from build123d import *

# Parameters (mm, degrees)
SKETCH1_W                      = 22.5
SKETCH1_H                      = 20
BOSS_EXTRUDE1_DEPTH            = 3.175
CBORE_FOR_M2_SHCS1_D           = 2.2
CBORE_FOR_M2_SHCS1_CBORE_D     = 4.4
CBORE_FOR_M2_SHCS1_CBORE_DEPTH = 2
TAP_DRILL_FOR_M2X0_4_TAP1_D    = 1.6
TAP_DRILL_FOR_M2X0_4_TAP2_D    = 1.6
FILLET1_SIZE                   = 1


with BuildPart() as part:
    # Sketch1 → Boss-Extrude1 (new body)
    with BuildSketch(Plane.XY):
        Rectangle(SKETCH1_W, SKETCH1_H)
    extrude(amount=BOSS_EXTRUDE1_DEPTH)

    # CBORE for M2 SHCS1 (through all)
    with Locations(Plane.XY.offset(3.175)):
        with Locations((4, 6), (-4, -6), (-4, 6), (4, -6)):
            CounterBoreHole(CBORE_FOR_M2_SHCS1_D / 2, CBORE_FOR_M2_SHCS1_CBORE_D / 2, CBORE_FOR_M2_SHCS1_CBORE_DEPTH)

    # Tap Drill for M2x0.4 Tap1 (through all)
    with Locations(Plane(origin=(0, 10, 0), x_dir=(1, 0, 0), z_dir=(0, 1, 0))):
        with Locations((8, -1.5875), (-8, -1.5875)):
            Hole(TAP_DRILL_FOR_M2X0_4_TAP1_D / 2)

    # Tap Drill for M2x0.4 Tap2 (through all)
    with Locations(Plane.XY.offset(3.175)):
        with Locations((0, 0), (-4.949747468, 0), (0, -4.949747468), (4.949747468, 0), (0, 4.949747468)):
            Hole(TAP_DRILL_FOR_M2X0_4_TAP2_D / 2)

    # Fillet1
    fillet1_edges = [part.edges().sort_by_distance(p)[0] for p in [
        (11.25, -10, 1.5875),
        (-11.25, -10, 1.5875),
        (-11.25, 10, 1.5875),
        (11.25, 10, 1.5875),
    ]]
    chamfer(fillet1_edges, length=FILLET1_SIZE)


solid = part.part
Geometry: final body of the model. Coordinates: model frame, mm. A direction names the side the tool comes from. Round coordinates to 2 decimals unless told otherwise and drop trailing zeros. Order: outer loops, then holes, each group sorted by start corner. A loop starts at its lowest first (then second) coordinate and runs counter-clockwise, first axis right, second up. Notation, with made-up numbers: (-32, -21) - (-18, -21) arc R34 cw to (-18, 15) - close; hole circle Ø1 at (35, 5.25). An arc over 180 degrees is marked (long way). Write each question's results on one line, items separated by ' | '.
Item 1: First-contact query: pin 1 Ø1.3 at (x, y) = (-3.5, 6.5) entering from +Z (3 decimals); pin 2 Ø1 at (x, y) = (4.95, 0) entering from +Z. Flat tips, straight axial feed; report the tip coordinate or a pass-through.
Completed:
pin 1: z = 1.175 | pin 2: through
Item 2: Section B-B, the plane x = -8. Return the cut outline in (y, z) (1 decimal).
Completed:
outline: (-10, 0) - (10, 0) - (10, 0.8) - (-10, 0.8) - close; (-10, 2.4) - (10, 2.4) - (10, 3.2) - (-10, 3.2) - close
Item 3: Reachability of faces 4 (the flat face through (10.76, -9.49, 1.57)), 5 (the cylindrical face through (-1.9, 6.66, 2.19)) from +Z, -Z, +X, -X, +Y, -Y: full face, straight path, thin tool, end or side. Return the list, or none.
Completed:
face 4: +Z, -Z, +X, -Y | face 5: +Z
Item 4: Section D-D, the plane x = -3.5. Return the cut outline in (y, z) (3 decimals), and give its area (3 significant figures).
Completed:
outline: (-10, 0) - (-6.98, 0) - (-6.98, 1.175) - (-8.142, 1.175) - (-8.142, 3.175) - (-10, 3.175) - close; (-5.02, 0) - (5.02, 0) - (5.02, 1.175) - (3.858, 1.175) - (3.858, 3.175) - (-3.858, 3.175) - (-3.858, 1.175) - (-5.02, 1.175) - close; (6.98, 0) - (10, 0) - (10, 3.175) - (8.142, 3.175) - (8.142, 1.175) - (6.98, 1.175) - close | area: 41.8 mm^2
Item 5: Section A-A, the plane y = 0. State how many separate pieces and enclosed holes the cut face has, and give its area (3 significant figures).
Completed:
separate pieces: 4 | enclosed holes: 2 | area: 52.2 mm^2
Item 6: Material intervals for line 1 along Y through (x, z) = (0, 0.9); line 2 along Y through (x, z) = (4, 0.3); line 3 along Y through (x, z) = (4, 2.65), sorted ascending. Write a range as [from, to].
Completed:
line 1: [-10, -5.75], [-4.15, -0.8], [0.8, 4.15], [5.75, 10] | line 2: [-10, -7.1], [-4.9, 4.9], [7.1, 10] | line 3: [-10, -8.2], [-3.8, 3.8], [8.2, 10]
Item 7: Mould query, pull axis Z, two halves, no side actions, for faces 1 (the flat face through (0, 2, 0)), 2 (the cylindrical face through (2.95, -5.67, 0.58)), 3 (the cylindrical face through (8.8, -0.1, 1.6)). Classes: pulls with the +Z half, pulls with the -Z half, needs draft (parallel to the pull), parting line crosses it, or undercut.
Completed:
face 1: pulls with the -Z half | face 2: needs draft | face 3: undercut
